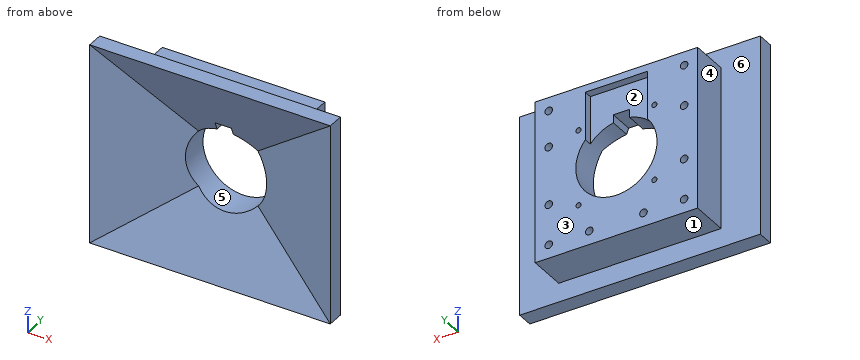
from build123d import *

# Parameters (mm, degrees)
SKETCH1_W           = 60
SKETCH1_H           = 60
BOSS_EXTRUDE1_DEPTH = 20
SKETCH10_W          = 15
SKETCH10_H          = 15
CUT_EXTRUDE4_DEPTH  = 8
SKETCH9_W           = 88.892246252
SKETCH9_H           = 74
SKETCH9_W_2         = 60
SKETCH9_H_2         = 60
BOSS_EXTRUDE4_DEPTH = 6
SKETCH2_R           = 15
CUT_EXTRUDE5_DEPTH  = 62.191975628
SKETCH11_R          = 0.95
CUT_EXTRUDE6_DEPTH  = 6
SKETCH12_W          = 23
SKETCH12_H          = 10.738639716
CUT_EXTRUDE7_DEPTH  = 3
SKETCH13_W          = 23
SKETCH13_H          = 7
CUT_EXTRUDE8_DEPTH  = 3
SKETCH14_R          = 1.4
CUT_EXTRUDE9_DEPTH  = 5
SKETCH15_W          = 6
SKETCH15_H          = 8
CUT_EXTRUDE10_DEPTH = 61.278170847


with BuildPart() as part:
    # Sketch1 → Boss-Extrude1 (new body)
    with BuildSketch(Plane(origin=(0, 0, 0), x_dir=(1, 0, 0), z_dir=(0, 1, 0))):
        Rectangle(SKETCH1_W, SKETCH1_H)
    extrude(amount=BOSS_EXTRUDE1_DEPTH)

    # Sketch10 → Cut-Extrude4 (cut)
    with BuildSketch(Plane(origin=(0, 20, 0), x_dir=(1, 0, 0), z_dir=(0, 1, 0))):
        Rectangle(SKETCH10_W, SKETCH10_H)
    extrude(amount=-CUT_EXTRUDE4_DEPTH, mode=Mode.SUBTRACT)

    # Sketch9 → Boss-Extrude4 (add)
    with BuildSketch(Plane.XZ):
        Rectangle(SKETCH9_W, SKETCH9_H)
        Rectangle(SKETCH9_W_2, SKETCH9_H_2, mode=Mode.SUBTRACT)
    extrude(amount=-BOSS_EXTRUDE4_DEPTH)

    # Cut-Loft2: read off the stored shape, not the designer's step
    # Cut-Loft2: loft between two sections, ruled curve by curve
    cut_loft2_from = [
        Edge.make_line((-7.5, 12, -7.5), (7.5, 12, -7.5)),
        Edge.make_line((7.5, 12, -7.5), (7.5, 12, 7.5)),
        Edge.make_line((-7.5, 12, 7.5), (-7.5, 12, -7.5)),
        Edge.make_line((7.5, 12, 7.5), (-7.5, 12, 7.5)),
    ]
    cut_loft2_to = [
        Edge.make_line((-44.446123126, 0, -37), (44.446123126, 0, -37)),
        Edge.make_line((44.446123126, 0, -37), (44.446123126, 0, 37)),
        Edge.make_line((-44.446123126, 0, 37), (-44.446123126, 0, -37)),
        Edge.make_line((44.446123126, 0, 37), (-44.446123126, 0, 37)),
    ]
    cut_loft2 = Solid(Shell([*[Face.make_surface_from_curves(cut_loft2_from[k], cut_loft2_to[k]) for k in range(4)], Face(Wire(cut_loft2_from)), Face(Wire(cut_loft2_to))]))
    add(cut_loft2, mode=Mode.SUBTRACT)

    # Sketch2 → Cut-Extrude5 (cut, through all)
    with BuildSketch(Plane(origin=(0, 20, 0), x_dir=(1, 0, 0), z_dir=(0, 1, 0))):
        with Locations(Location((0, 0, 0), (0, 0, 270))):
            Circle(SKETCH2_R)
    extrude(amount=-CUT_EXTRUDE5_DEPTH, mode=Mode.SUBTRACT)

    # Sketch11 → Cut-Extrude6 (cut)
    with BuildSketch(Plane(origin=(0, 20, 0), x_dir=(1, 0, 0), z_dir=(0, 1, 0))):
        with Locations(Location((-14, 14, 0), (0, 0, 270))):
            Circle(SKETCH11_R)
        with Locations(Location((14, 14, 0), (0, 0, 270))):
            Circle(SKETCH11_R)
        with Locations(Location((14, -14, 0), (0, 0, 270))):
            Circle(SKETCH11_R)
        with Locations(Location((-14, -14, 0), (0, 0, 270))):
            Circle(SKETCH11_R)
    extrude(amount=-CUT_EXTRUDE6_DEPTH, mode=Mode.SUBTRACT)

    # Sketch12 → Cut-Extrude7 (cut)
    with BuildSketch(Plane(origin=(0, 20, 0), x_dir=(1, 0, 0), z_dir=(0, 1, 0))):
        with Locations((0, -15)):
            Rectangle(SKETCH12_W, SKETCH12_H)
    extrude(amount=-CUT_EXTRUDE7_DEPTH, mode=Mode.SUBTRACT)

    # Sketch13 → Cut-Extrude8 (cut)
    with BuildSketch(Plane(origin=(0, 20, 0), x_dir=(1, 0, 0), z_dir=(0, 1, 0))):
        with Locations((0, -23.869319858)):
            Rectangle(SKETCH13_W, SKETCH13_H)
    extrude(amount=-CUT_EXTRUDE8_DEPTH, mode=Mode.SUBTRACT)

    # Sketch14 → Cut-Extrude9 (cut)
    with BuildSketch(Plane(origin=(0, 20, 0), x_dir=(1, 0, 0), z_dir=(0, 1, 0))):
        with Locations(Location((-25, 25, 0), (0, 0, 270))):
            Circle(SKETCH14_R)
        with Locations(Location((25, 25, 0), (0, 0, 270))):
            Circle(SKETCH14_R)
        with Locations(Location((25, -25, 0), (0, 0, 270))):
            Circle(SKETCH14_R)
        with Locations(Location((-25, -25, 0), (0, 0, 270))):
            Circle(SKETCH14_R)
        with Locations(Location((-10, 25, 0), (0, 0, 270))):
            Circle(SKETCH14_R)
        with Locations(Location((10, 25, 0), (0, 0, 270))):
            Circle(SKETCH14_R)
        with Locations(Location((-25, 10, 0), (0, 0, 270))):
            Circle(SKETCH14_R)
        with Locations(Location((-25, -10, 0), (0, 0, 270))):
            Circle(SKETCH14_R)
        with Locations(Location((25, 10, 0), (0, 0, 270))):
            Circle(SKETCH14_R)
        with Locations(Location((25, -11.506341958, 0), (0, 0, 270))):
            Circle(SKETCH14_R)
    extrude(amount=-CUT_EXTRUDE9_DEPTH, mode=Mode.SUBTRACT)

    # Sketch15 → Cut-Extrude10 (cut, through all)
    with BuildSketch(Plane(origin=(0, 17, 0), x_dir=(1, 0, 0), z_dir=(0, 1, 0))):
        with Locations((0, -13.684659929)):
            Rectangle(SKETCH15_W, SKETCH15_H)
    extrude(amount=-CUT_EXTRUDE10_DEPTH, mode=Mode.SUBTRACT)


solid = part.part
Check sheet for the modelled part. Datum: model origin and axes. Units: mm. Face numbers are marked on the shaded views. A direction names the side the tool comes from. Give positions to 0.01 mm unless a question says otherwise; leave off trailing zeros. Answer as a JSON object with one key per item and string values. Group by question number.
Q1. Material ranges on line 1 along X through (y, z) = (18.4, 25); line 2 along X through (y, z) = (16.2, -25); line 3 along X through (y, z) = (18.05, 14), recorded low to high. Write a range as [from, to].
Q2. Go/stop test with flat-tipped pins: P1, Ø0.9, axis at x = -14, z = 14, coming from the +Y side; P2, Ø4, axis at x = 6.5, y = 12, coming from the +Z side; P3, Ø5, axis at x = 1, y = 14, coming from the -Z side. Record where each tip stops, or that it passes through.
Q3. Release check for a two-part mould opening along X. For the marked faces 4, 5 and 6 record: released by +X, released by -X, zero draft, split by the parting line, or undercut.
Q4. Access from +Z, -Z, +X, -X, +Y, -Y to the whole of each face (thin tool, end or side, straight path). Record for the marked faces 1, 2 and 3.
Evaluation:
{
 "1": {"line 1": "x = [-30, -26.4], [-23.6, -11.5], [11.5, 23.6], [26.4, 30]", "line 2": "x = [-30, -26.4], [-23.6, -11.4], [-8.6, 8.6], [11.4, 23.6], [26.4, 30]", "line 3": "x = [-30, -14.95], [-13.05, -11.5], [11.5, 13.05], [14.95, 30]"},
 "2": {"P1": "stops at y = 14", "P2": "stops at z = 30", "P3": "stops at z = -30"},
 "3": {"face 4": "released by -X", "face 5": "undercut", "face 6": "zero draft"},
 "4": {"face 1": "-Z, +X, -X, +Y", "face 2": "+Y", "face 3": "+Z, -Z, +X, -X, +Y"}
}
